```python
from build123d import *

# Parameters (mm, degrees)
SKETCH1_W               = 52
SKETCH1_H               = 56
SKETCH1_R               = 2.95
BOSS_EXTRUDE1_DEPTH     = 10
CUT_EXTRUDE1_DEPTH      = 78.071395472
CUT_EXTRUDE1_DEPTH_BACK = 5
SKETCH2_R               = 4.5
BOSS_EXTRUDE2_START     = -14.75
SKETCH3_W               = 5
SKETCH3_H               = 20
BOSS_EXTRUDE2_DEPTH     = 22.5
CUT_EXTRUDE2_REACH      = 69.337
CHAMFER1_SIZE           = 14.75
CHAMFER2_SIZE           = 2.5


with BuildPart() as part:
    # Sketch1 → Boss-Extrude1 (new body)
    with BuildSketch(Plane(origin=(0, 0, 0), x_dir=(1, 0, 0), z_dir=(0, 1, 0))):
        with Locations((26, 28)):
            Rectangle(SKETCH1_W, SKETCH1_H)
        with Locations(Location((10, 46, 0), (0, 0, 270))):
            Circle(SKETCH1_R, mode=Mode.SUBTRACT)
        with Locations(Location((42, 46, 0), (0, 0, 270))):
            Circle(SKETCH1_R, mode=Mode.SUBTRACT)
        with Locations(Location((42, 10, 0), (0, 0, 270))):
            Circle(SKETCH1_R, mode=Mode.SUBTRACT)
        with Locations(Location((10, 10, 0), (0, 0, 270))):
            Circle(SKETCH1_R, mode=Mode.SUBTRACT)
    extrude(amount=BOSS_EXTRUDE1_DEPTH)

    # Sketch2 → Cut-Extrude1 (cut, two sides: drawn at the far end of the back side and taken through both)
    with BuildSketch(Plane(origin=(0, 10, 0), x_dir=(1, 0, 0), z_dir=(0, 1, 0)).offset(-CUT_EXTRUDE1_DEPTH_BACK)):
        with Locations(Location((10, 10, 0), (0, 0, 90))):
            Circle(SKETCH2_R)
        with Locations(Location((42, 10, 0), (0, 0, 90))):
            Circle(SKETCH2_R)
        with Locations(Location((42, 46, 0), (0, 0, 90))):
            Circle(SKETCH2_R)
        with Locations(Location((10, 46, 0), (0, 0, 90))):
            Circle(SKETCH2_R)
    extrude(amount=CUT_EXTRUDE1_DEPTH + CUT_EXTRUDE1_DEPTH_BACK, mode=Mode.SUBTRACT)

    # Sketch3 → Boss-Extrude2 (add)
    with BuildSketch(Plane(origin=(52, 0, 0), x_dir=(0, 0, -1), z_dir=(1, 0, 0)).offset(BOSS_EXTRUDE2_START)):
        with Locations((28, 20)):
            Rectangle(SKETCH3_W, SKETCH3_H)
        with Locations((53.5, 20)):
            Rectangle(SKETCH3_W, SKETCH3_H)
    extrude(amount=-BOSS_EXTRUDE2_DEPTH)

    # Cut-Extrude2: up to this face of the body (flat: up to its plane)
    cut_extrude2_end = Plane(part.part.faces().sort_by_distance((26, 11.958762887, -56))[0])
    # Sketch4 → Cut-Extrude2 (cut, up to the picked face)
    with BuildSketch(Plane.XY.offset(-25.5), mode=Mode.PRIVATE) as cut_extrude2_sk1:
        with BuildLine():
            Line((22.875, 22.5), (22.875, 17.5))
            ThreePointArc((22.875, 17.5), (20.375, 15), (17.875, 17.5))
            Line((17.875, 17.5), (17.875, 22.5))
            ThreePointArc((17.875, 22.5), (20.375, 25), (22.875, 22.5))
        make_face()
    cut_extrude2_tool1 = split(extrude(cut_extrude2_sk1.sketch, amount=-CUT_EXTRUDE2_REACH, mode=Mode.PRIVATE), bisect_by=cut_extrude2_end, keep=Keep.BOTH, mode=Mode.PRIVATE)
    # Sketch4 → Cut-Extrude2 (cut, up to the picked face)
    with BuildSketch(Plane.XY.offset(-25.5), mode=Mode.PRIVATE) as cut_extrude2_sk2:
        with BuildLine():
            Line((34.125, 22.5), (34.125, 17.5))
            ThreePointArc((34.125, 17.5), (31.625, 15), (29.125, 17.5))
            Line((29.125, 17.5), (29.125, 22.5))
            ThreePointArc((29.125, 22.5), (31.625, 25), (34.125, 22.5))
        make_face()
    cut_extrude2_tool2 = split(extrude(cut_extrude2_sk2.sketch, amount=-CUT_EXTRUDE2_REACH, mode=Mode.PRIVATE), bisect_by=cut_extrude2_end, keep=Keep.BOTH, mode=Mode.PRIVATE)
    add(cut_extrude2_tool1.solids().sort_by(Axis((20.375, 20, -25.5), (0, 0, -1)))[0], mode=Mode.SUBTRACT)
    add(cut_extrude2_tool2.solids().sort_by(Axis((31.625, 20, -25.5), (0, 0, -1)))[0], mode=Mode.SUBTRACT)

    # Chamfer1
    chamfer1_edges = [part.edges().sort_by_distance(p)[0] for p in [
        (37.25, 10, -53.5),
        (37.25, 10, -28),
        (14.75, 10, -53.5),
        (14.75, 10, -28),
    ]]
    chamfer(chamfer1_edges, length=CHAMFER1_SIZE - 0.0001)  # a hair under: the kernel refuses the full size

    # Chamfer2
    chamfer2_edges = [part.edges().sort_by_distance(p)[0] for p in [
        (26, 10, -25.5),
    ]]
    chamfer(chamfer2_edges, length=CHAMFER2_SIZE)


solid = part.part
```
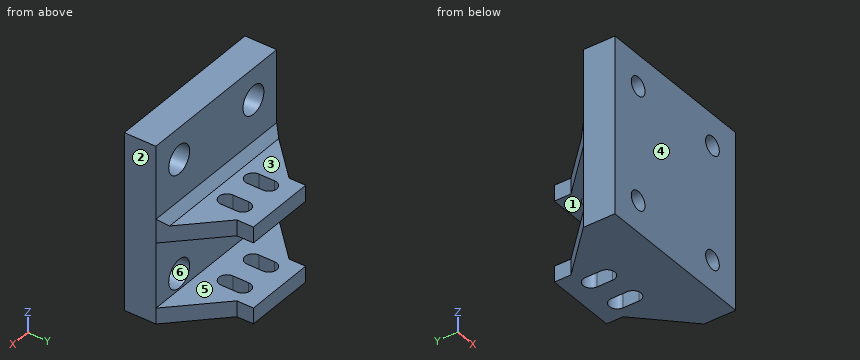
CAD build for the part. Positions are in the model's coordinates, mm. Face numbers are marked on the shaded views. A direction names the side the tool comes from. Round coordinates to 2 decimals unless told otherwise and drop trailing zeros. Loops run counter-clockwise (first coordinate to the right, second up) from the corner with the lowest first, then second, coordinate; pieces in that order, holes last. Notation, with made-up numbers: M -31,71.25 L -15,71.25 A28 cw -15,90.25 Z; hole C 16.25,72.25 d7. An arc over 180 degrees is marked long. Return JSON: item names as keys, results as strings. Group by question number.
(1) Drop flat-ended pins along their axis: P1, Ø2.5, axis at y = 27.5, z = -54.5, coming from the +X side; P2, Ø5.5, axis at x = 42, z = -10, coming from the +Y side; P3, Ø4, axis at y = 21, z = -54, coming from the +X side; P4, Ø5, axis at x = 28, y = 26.5, coming from the +Z side. Give the stop position or say it passes through.
(2) Tool access for the marked faces 4, 5 and 6: list every direction of +Z, -Z, +X, -X, +Y, -Y with a clear straight run to the whole face (end or side of a thin tool).
(3) Saw through at D-D, the plane x = 44. List the corners of the cut face in (y, z), and give its area (3 significant figures).
(4) Saw through at B-B, the plane y = 27. List the corners of the cut face in (x, z).
(5) Saw through at C-C, the plane y = 2.25. List the corners of the cut face in (x, z).
(6) Mould opens along Z. For the marked faces 1, 2 and 3 say: +Z half, -Z half, draft (parallel to the pull), parting line (faces both ways), or undercut.
(7) Wall check: probe 1 along X at (y, z) = (2.3, -10); probe 2 along Z at (x, y) = (42, 8.75); probe 3 along X at (y, z) = (7.65, -46). Give the ranges that are in metal, low to high. Write a range as [from, to].
(8) Saw through at A-A, the plane z = -10. List the corners of the cut face in (x, y), and give its area (3 significant figures).
Answer list:
{
 "1": {"P1": "x = 37.25", "P2": "through", "P3": "x = 43", "P4": "z = -25.5"},
 "2": {"face 4": "+Z, -Z, +X, -X, -Y", "face 5": "+X, -X, +Y", "face 6": "+Y"},
 "3": {"outline": "M 0,-56 L 18,-56 L 18,-51 L 10,-51 L 10,-50.03 L 5,-50.03 L 5,-48.17 L 0,-48.17 Z; M 0,-43.83 L 5,-43.83 L 5,-41.97 L 10,-41.97 L 10,-30.5 L 18,-30.5 L 18,-25.5 L 12.5,-25.5 L 10,-23 L 10,-14.03 L 5,-14.03 L 5,-12.17 L 0,-12.17 Z; M 0,-7.83 L 5,-7.83 L 5,-5.97 L 10,-5.97 L 10,0 L 0,0 Z", "area": "519 mm2"},
 "4": {"outline": "M 14.75,-56 L 37.25,-56 L 37.25,-51 L 14.75,-51 Z; M 14.75,-30.5 L 37.25,-30.5 L 37.25,-25.5 L 14.75,-25.5 Z"},
 "5": {"outline": "M 0,-56 L 52,-56 L 52,0 L 0,0 Z; hole C 10,-46 d5.9; hole C 10,-10 d5.9; hole C 42,-46 d5.9; hole C 42,-10 d5.9"},
 "6": {"face 1": "undercut", "face 2": "draft", "face 3": "+Z half"},
 "7": {"probe 1": "[0, 7.05], [12.95, 39.05], [44.95, 52]", "probe 2": "[-56, -50.5], [-41.5, -14.5], [-5.5, 0]", "probe 3": "[0, 5.5], [14.5, 37.5], [46.5, 52]"},
 "8": {"outline": "M 0,0 L 7.05,0 L 7.05,5 L 5.5,5 L 5.5,10 L 0,10 Z; M 12.95,0 L 39.05,0 L 39.05,5 L 37.5,5 L 37.5,10 L 14.5,10 L 14.5,5 L 12.95,5 Z; M 44.95,0 L 52,0 L 52,10 L 46.5,10 L 46.5,5 L 44.95,5 Z", "area": "371 mm2"}
}
